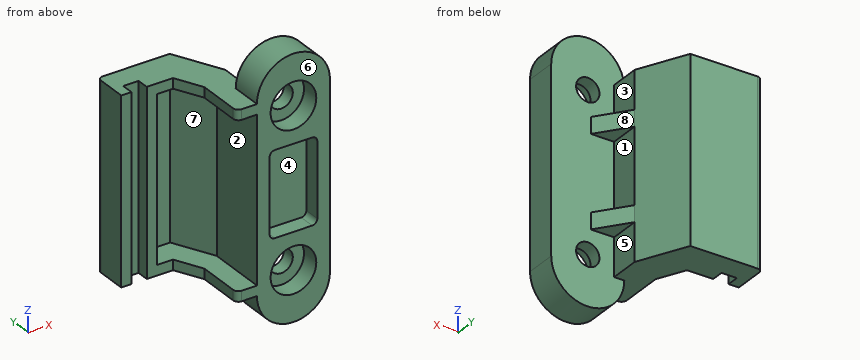
```python
from build123d import *

# Parameters (mm, degrees)
EXTRUSION1_DEPTH                                  = 18.1
COQUE1_START                                      = 1
COQUE1_DEPTH                                      = 16.1
EXTRUSION2_DEPTH                                  = 3.1
ESQUISSE3_W                                       = 6.2
ESQUISSE3_H                                       = 18.1
EXTRUSION3_DEPTH                                  = 2.1
CHAMBRAGE_POUR_VIS_T_TE_HEXAGONALE_M2_D           = 2.3
CHAMBRAGE_POUR_VIS_T_TE_HEXAGONALE_M2_CBORE_D     = 4.5
CHAMBRAGE_POUR_VIS_T_TE_HEXAGONALE_M2_CBORE_DEPTH = 1.8
ENL_V_MAT_EXTRU_1_DEPTH                           = 1.6
EXTRUSION4_DEPTH                                  = 1.6
R_P_TITION_LIN_AIRE1_COUNT                        = 2
R_P_TITION_LIN_AIRE1_PITCH                        = 9


# Read off the part's stored shape, not the designer's step: Coque1
with BuildPart() as part:
    # Esquisse1 → Extrusion1 (new body)
    with BuildSketch(Plane.XY):
        with BuildLine():
            Line((0.5, 0), (9.2, 0))
            Line((9.2, 0), (9.2, 3.1))
            Line((9.2, 3.1), (3, 3.1))
            Line((3, 3.1), (3, 6.1))
            Line((3, 6.1), (0.698275932, 10.81853434))
            Line((0.698275932, 10.81853434), (-5.901724068, 10.81853434))
            ThreePointArc((-5.901724068, 10.81853434), (-6.255277459, 10.67208773), (-6.401724068, 10.31853434))
            Line((-6.401724068, 10.31853434), (-6.401724068, 7.36853434))
            Line((-6.401724068, 7.36853434), (-5.401724068, 7.36853434))
            Line((-5.401724068, 7.36853434), (-5.401724068, 8.56853434))
            Line((-5.401724068, 8.56853434), (-3.884726415, 8.56853434))
            Line((-3.884726415, 8.56853434), (-3.884726415, 7.36853434))
            Line((-3.884726415, 7.36853434), (-1.301724068, 7.36853434))
            Line((-1.301724068, 7.36853434), (0, 4.7))
            Line((0, 4.7), (0, 0.5))
            ThreePointArc((0, 0.5), (0.146446609, 0.146446609), (0.5, 0))
        make_face()
    extrude(amount=EXTRUSION1_DEPTH)

    # Coque1 outline → Coque1 (cut)
    with BuildSketch(Plane.XY.offset(COQUE1_START)):
        with BuildLine():
            Line((-5.401724068, 9.81853434), (-5.401724068, 9.56853434))
            Line((-5.401724068, 9.56853434), (-2.884726415, 9.56853434))
            Line((-2.884726415, 9.56853434), (-2.884726415, 7.36853434))
            Line((-2.884726415, 7.36853434), (-1.301724068, 7.36853434))
            Line((-1.301724068, 7.36853434), (0, 4.7))
            Line((0, 4.7), (0, 0.5))
            ThreePointArc((0, 0.5), (0.146446609, 0.146446609), (0.5, 0))
            Line((0.5, 0), (8.2, 0))
            Line((8.2, 0), (8.2, 2.1))
            Line((8.2, 2.1), (2, 2.1))
            Line((2, 2.1), (2, 5.869101054))
            Line((2, 5.869101054), (0.073447178, 9.81853434))
            Line((0.073447178, 9.81853434), (-5.401724068, 9.81853434))
        make_face()
    extrude(amount=COQUE1_DEPTH, mode=Mode.SUBTRACT)

    # Esquisse2 → Extrusion2 (add)
    with BuildSketch(Plane(origin=(0, 3.1, 0), x_dir=(-1, 0, 0), z_dir=(0, 1, 0))):
        with BuildLine():
            Line((-9.2, 0), (-2, 0))
            ThreePointArc((-2, 0), (-5.6, -3.6), (-9.2, 0))
        make_face()
        with BuildLine():
            Line((-9.2, 18.1), (-2, 18.1))
            ThreePointArc((-2, 18.1), (-5.6, 21.7), (-9.2, 18.1))
        make_face()
    extrude(amount=-EXTRUSION2_DEPTH)

    # Esquisse3 → Extrusion3 (add)
    with BuildSketch(Plane.XZ):
        with Locations((5.1, 9.05)):
            Rectangle(ESQUISSE3_W, ESQUISSE3_H)
    extrude(amount=-EXTRUSION3_DEPTH)

    # Chambrage pour vis à tête hexagonale M2.51 (through all)
    with Locations(Plane.XZ):
        with Locations((5.6, 1.3), (5.6, 16.8)):
            CounterBoreHole(CHAMBRAGE_POUR_VIS_T_TE_HEXAGONALE_M2_D / 2, CHAMBRAGE_POUR_VIS_T_TE_HEXAGONALE_M2_CBORE_D / 2, CHAMBRAGE_POUR_VIS_T_TE_HEXAGONALE_M2_CBORE_DEPTH)

    # Esquisse6 → Enlèv. mat.-Extru.1 (cut)
    with BuildSketch(Plane.XZ):
        with BuildLine():
            Line((3.75, 4.9), (7.45, 4.9))
            ThreePointArc((7.45, 4.9), (7.803553391, 5.046446609), (7.95, 5.4))
            Line((7.95, 5.4), (7.95, 12.7))
            ThreePointArc((7.95, 12.7), (7.803553391, 13.053553391), (7.45, 13.2))
            Line((7.45, 13.2), (3.75, 13.2))
            ThreePointArc((3.75, 13.2), (3.396446609, 13.053553391), (3.25, 12.7))
            Line((3.25, 12.7), (3.25, 5.4))
            ThreePointArc((3.25, 5.4), (3.396446609, 5.046446609), (3.75, 4.9))
        make_face()
    extrude(amount=-ENL_V_MAT_EXTRU_1_DEPTH, mode=Mode.SUBTRACT)

    # Esquisse7 → Extrusion4 (add)
    with BuildSketch(Plane.XY.offset(14.35)):
        Polygon((3, 6.1), (5.3, 3.1), (3, 3.1), align=None)
    extrusion4 = extrude(amount=-EXTRUSION4_DEPTH)

    # Répétition linéaire1: Extrusion4 ×2
    with Locations(*[(0, 0, -i * R_P_TITION_LIN_AIRE1_PITCH) for i in range(1, R_P_TITION_LIN_AIRE1_COUNT)]):
        add(extrusion4)


solid = part.part
```
Part model, mm, in its own coordinate system. Face numbers are marked on the shaded views. A direction names the side the tool comes from. Coordinates: 2 decimals unless noted, no trailing zeros. Order: outer loops, then holes, each group sorted by start corner. A loop starts at its lowest first (then second) coordinate and runs counter-clockwise, first axis right, second up. Notation, with made-up numbers: (-26, 24.25) - (-11, 24.25) arc R3 cw to (-11, 28.25) - close; hole circle Ø9 at (73.5, 25). An arc over 180 degrees is marked (long way). Return JSON: item names as keys, results as strings. Group by question number.
Item 1: Pull direction X, two halves, no side cores. Call the marked faces 6, 7 and 8: pulls with the +X half, pulls with the -X half, needs draft (parallel to the pull), parting line crosses it, or undercut.
Item 2: Cut at C-C (x = -2.25). List the corners of the cut face in (y, z), plus the area to 3 significant figures.
Item 3: Drill centre lines: probe 1 along Z at (x, y) = (5.6, 1.25); probe 2 along Z at (x, y) = (5.6, 2.3); probe 3 along X at (y, z) = (0.75, 12.5). Where is each one in solid material? Low to high. Write a range as from..to.
Item 4: Cut at A-A (z = 16.8). List the corners of the cut face in (x, y), plus the area to 3 significant figures.
Item 5: Cut at B-B (x = 5.6). List the corners of the cut face in (y, z), plus the area to 3 significant figures.
Item 6: Which spindle directions (+Z, -Z, +X, -X, +Y, -Y) get a long thin tool onto all of the face, cutting with end or side? Do the marked faces 1, 2, 3, 4 and 5. Say none if no direction does.
Item 7: Pin check, flat tips, straight feed: pin 1 (6 mm diameter, centred on x = -3, y = 6, fed in from +Z); pin 2 (1.8 mm diameter, centred on y = 8.5, z = 7, fed in from +X); pin 3 (1 mm diameter, centred on y = 6, z = 10, fed in from +X). Stop position of each tip, or through.
Item 8: Cut at D-D (z = 14). List the corners of the cut face in (x, y), plus the area to 3 significant figures.
Check values:
{
 "1": {"face 6": "needs draft", "face 7": "undercut", "face 8": "pulls with the +X half"},
 "2": {"outline": "(7.37, 0) - (10.82, 0) - (10.82, 18.1) - (7.37, 18.1) - (7.37, 17.1) - (9.82, 17.1) - (9.82, 1) - (7.37, 1) - close", "area": "23.0 mm2"},
 "3": {"probe 1": "z = -3.6..-0.95, 3.55..4.9, 13.2..14.55, 19.05..21.7", "probe 2": "z = -3.6..0.15, 2.45..15.65, 17.95..21.7", "probe 3": "x = 2..3.25, 7.95..9.2"},
 "4": {"outline": "(-6.4, 7.37) - (-5.4, 7.37) - (-5.4, 8.57) - (-3.88, 8.57) - (-3.88, 7.37) - (-2.88, 7.37) - (-2.88, 9.57) - (-5.4, 9.57) - (-5.4, 9.82) - (0.07, 9.82) - (2, 5.87) - (2, 0) - (3.35, 0) - (3.35, 1.8) - (4.45, 1.8) - (4.45, 3.1) - (3, 3.1) - (3, 6.1) - (0.7, 10.82) - (-5.9, 10.82) arc R0.5 ccw to (-6.4, 10.32) - close; (6.75, 1.8) - (7.85, 1.8) - (7.85, 0) - (9.2, 0) - (9.2, 3.1) - (6.75, 3.1) - close", "area": "31.8 mm2"},
 "5": {"outline": "(0, -3.6) - (3.1, -3.6) - (3.1, 0.15) - (1.8, 0.15) - (1.8, -0.95) - (0, -0.95) - close; (0, 3.55) - (1.8, 3.55) - (1.8, 2.45) - (3.1, 2.45) - (3.1, 15.65) - (1.8, 15.65) - (1.8, 14.55) - (0, 14.55) - (0, 13.2) - (1.6, 13.2) - (1.6, 4.9) - (0, 4.9) - close; (0, 19.05) - (1.8, 19.05) - (1.8, 17.95) - (3.1, 17.95) - (3.1, 21.7) - (0, 21.7) - close", "area": "43.0 mm2"},
 "6": {"face 1": "+X, +Y", "face 2": "-X, -Y", "face 3": "+Z, +X, +Y", "face 4": "-Y", "face 5": "-Z, +X, +Y"},
 "7": {"pin 1": "stops at z = 18.1", "pin 2": "stops at x = 2.27", "pin 3": "stops at x = 3"},
 "8": {"outline": "(-6.4, 7.37) - (-5.4, 7.37) - (-5.4, 8.57) - (-3.88, 8.57) - (-3.88, 7.37) - (-2.88, 7.37) - (-2.88, 9.57) - (-5.4, 9.57) - (-5.4, 9.82) - (0.07, 9.82) - (2, 5.87) - (2, 0) - (9.2, 0) - (9.2, 3.1) - (5.3, 3.1) - (3, 6.1) - (0.7, 10.82) - (-5.9, 10.82) arc R0.5 ccw to (-6.4, 10.32) - close", "area": "46.4 mm2"}
}
